The listing builds one solid part. Answer for the finished solid, in the listing's coordinates (mm). A direction names the side the tool comes from. Round coordinates to 2 decimals unless told otherwise and drop trailing zeros. Order: outer loops, then holes, each group sorted by start corner. A loop starts at its lowest first (then second) coordinate and runs counter-clockwise, first axis right, second up. Notation, with made-up numbers: (17.5, -26.5) - (64.5, -26.5) arc R26 cw to (64.5, -10.5) - close; hole circle Ø7 at (-5, 6.5). An arc over 180 degrees is marked (long way). One line per item, written item: value. Start each with the question number.
1. Flat-ended cylindrical pins translate along their axes: P1, Ø5, axis at x = -8, z = -16, coming from the +Y side (3 decimals); P2, Ø3, axis at x = -0.5, z = -17, coming from the -Y side; P3, Ø12, axis at x = -16, z = -20.5, coming from the -Y side; P4, Ø1, axis at y = -24, z = -27.5, coming from the +X side. Find the tip coordinate at first contact, or state that the pin passes through.
2. Section C-C, the plane z = -25 is taken. Give the vertices of the cut face in (x, y).
3. Straight lines are drawn through the part: line 1 (X direction, y = -24.5, z = -15.5); line 2 (Y direction, x = 30, z = -15); line 3 (Z direction, x = 1, y = -14). For each, find the intervals that lie inside material, in ascending order.
4. Section D-D, the plane z = -10.5 is taken. Give the vertices of the cut face in (x, y).
5. Section B-B, the plane y = 0 is taken. Give the vertices of the cut face in (x, z).
6. Section A-A, the plane x = -2 is taken. Give the vertices of the cut face in (y, z).
7. For a pull along Y with two mould halves and no side action, classify faces 1 (the cylindrical face through (27.675, -9.693, -10.846)), 2 (the flat face through (-0.5, -6.2, 0)), 3 (the cylindrical face through (-0.78, -5.95, -15.78)), 4 (the flat face through (-1, -13.016, -15)) as released by +Y, released by -Y, zero draft, split by the parting line, or undercut.
8. A tool of negligible diameter and unlimited length cuts with its end or side. For faces 5 (the flat face through (-30, -10, -11)), 6 (the flat face through (7.967, -24, -16)), 7 (the flat face through (24, 6, -22)), 8 (the cylindrical face through (-0.448, -21.128, -12.426)), from which of +Z, -Z, +X, -X, +Y, -Y can it reach the whole face along a straight path? Write none if from no direction.
from build123d import *

# Parameters (mm, degrees)
SKETCH1_R           = 6
BOSS_EXTRUDE1_DEPTH = 22
SKETCH3_R           = 3
CUT_EXTRUDE2_DEPTH  = 22
SKETCH4_R           = 6
BOSS_EXTRUDE2_DEPTH = 10
SKETCH5_R           = 3
CUT_EXTRUDE3_DEPTH  = 16


with BuildPart() as part:
    # Sketch1 → Boss-Extrude1 (new body)
    with BuildSketch(Plane.XY):
        with BuildLine():
            ThreePointArc((12.250598906, 10.291881579), (6.757584433, 14.502932553), (0, 16))
            ThreePointArc((0, 16), (-6.42506456, 14.653277633), (-11.768531852, 10.839818174))
            Line((-11.768531852, 10.839818174), (-13.649705535, 8.347786462))
            Line((-13.649705535, 8.347786462), (-26.599782678, -8.807462524))
            ThreePointArc((-26.599782678, -8.807462524), (-27.656705011, -9.685366602), (-28.994167614, -10))
            Line((-28.994167614, -10), (-32.032992561, -10))
            Line((-32.032992561, -10), (-32.032992561, -20.01649628))
            Line((-32.032992561, -20.01649628), (-27.5, -20.01649628))
            Line((-27.5, -20.01649628), (-8.032992561, -20.01649628))
            Line((-8.032992561, -20.01649628), (-8.032992561, -29.01649628))
            Line((-8.032992561, -29.01649628), (-0.032992561, -29.01649628))
            Line((-0.032992561, -29.01649628), (7.967007439, -29.01649628))
            Line((7.967007439, -29.01649628), (7.967007439, -20.01649628))
            Line((7.967007439, -20.01649628), (27.5, -20.01649628))
            Line((27.5, -20.01649628), (31.967007439, -20.01649628))
            Line((31.967007439, -20.01649628), (31.967007439, -10))
            Line((31.967007439, -10), (28.998198652, -10))
            ThreePointArc((28.998198652, -10), (27.65784727, -9.683925888), (26.599929469, -8.802305447))
            Line((26.599929469, -8.802305447), (13.293285189, 8.904412888))
            Line((13.293285189, 8.904412888), (12.250598906, 10.291881579))
        make_face()
        Circle(SKETCH1_R, mode=Mode.SUBTRACT)
    extrude(amount=-BOSS_EXTRUDE1_DEPTH)

    # Sketch3 → Cut-Extrude2 (cut)
    with BuildSketch(Plane(origin=(0, 0, 0), x_dir=(1, 0, 0), z_dir=(0, 1, 0))):
        with Locations(Location((0, 11.125223176, 0), (0, 0, 90))):
            Circle(SKETCH3_R)
    extrude(amount=CUT_EXTRUDE2_DEPTH, mode=Mode.SUBTRACT)

    # Sketch4 → Boss-Extrude2 (add)
    # profile 1 of 3: a face of its own
    with BuildSketch(Plane(origin=(0, 0, -22), x_dir=(-1, 0, 0), z_dir=(0, 0, -1))):
        with BuildLine():
            ThreePointArc((-12.250598906, 10.291881579), (-6.922536855, 14.424925771), (-0.364905179, 15.99583834))
            Line((-0.364905179, 15.99583834), (-32.361209339, 15.509505054))
            Line((-32.361209339, 15.509505054), (-31.967007439, -10))
            Line((-31.967007439, -10), (-28.998198652, -10))
            ThreePointArc((-28.998198652, -10), (-27.65784727, -9.683925888), (-26.599929469, -8.802305447))
            Line((-26.599929469, -8.802305447), (-12.250598906, 10.291881579))
        make_face()
    # profile 2 of 3: a face of its own
    with BuildSketch(Plane(origin=(0, 0, -22), x_dir=(-1, 0, 0), z_dir=(0, 0, -1))):
        with BuildLine():
            Line((31.626771502, 16.725648698), (-0.364905179, 15.99583834))
            ThreePointArc((-0.364905179, 15.99583834), (6.257540356, 14.725596378), (11.768531852, 10.839818174))
            Line((11.768531852, 10.839818174), (26.599782678, -8.807462524))
            ThreePointArc((26.599782678, -8.807462524), (27.656705011, -9.685366602), (28.994167614, -10))
            Line((28.994167614, -10), (32.032992561, -10))
            Line((32.032992561, -10), (31.626771502, 16.725648698))
        make_face()
    # profile 3 of 3: a face of its own
    with BuildSketch(Plane(origin=(0, 0, -22), x_dir=(-1, 0, 0), z_dir=(0, 0, -1))):
        with BuildLine():
            Line((32.032992561, -10), (28.994167614, -10))
            ThreePointArc((28.994167614, -10), (27.656705011, -9.685366602), (26.599782678, -8.807462524))
            Line((26.599782678, -8.807462524), (11.768531852, 10.839818174))
            ThreePointArc((11.768531852, 10.839818174), (-0.364905179, 15.99583834), (-12.250598906, 10.291881579))
            Line((-12.250598906, 10.291881579), (-26.599929469, -8.802305447))
            ThreePointArc((-26.599929469, -8.802305447), (-27.65784727, -9.683925888), (-28.998198652, -10))
            Line((-28.998198652, -10), (-31.967007439, -10))
            Line((-31.967007439, -10), (-31.967007439, -20.01649628))
            Line((-31.967007439, -20.01649628), (-7.967007439, -20.01649628))
            Line((-7.967007439, -20.01649628), (-7.967007439, -29.01649628))
            Line((-7.967007439, -29.01649628), (8.032992561, -29.01649628))
            Line((8.032992561, -29.01649628), (8.032992561, -20.01649628))
            Line((8.032992561, -20.01649628), (32.032992561, -20.01649628))
            Line((32.032992561, -20.01649628), (32.032992561, -10))
        make_face()
        with Locations(Location((0, 0, 0), (0, 0, 180))):
            Circle(SKETCH4_R, mode=Mode.SUBTRACT)
    extrude(amount=BOSS_EXTRUDE2_DEPTH)

    # Sketch5 → Cut-Extrude3 (cut)
    with BuildSketch(Plane.XZ.offset(29.01649628)):
        with Locations(Location((-0.579448602, -15.423300258, 0), (0, 0, 270))):
            Circle(SKETCH5_R)
    extrude(amount=-CUT_EXTRUDE3_DEPTH, mode=Mode.SUBTRACT)


solid = part.part
Answer list:
1. P1: stops at y = 15.025
1. P2: stops at y = -29.02
1. P3: stops at y = -20.02
1. P4: stops at x = 7.97
2. outline: (-32.03, -20.02) - (-8.03, -20.02) - (-8.03, -29.02) - (7.97, -29.02) - (7.97, -20.02) - (31.97, -20.02) - (31.97, -10) - (32.36, 15.51) - (0.36, 16) - (-31.63, 16.73) - (-32.03, -10) - close; hole circle Ø12 at (0, 0)
3. line 1: x = -8.03 to -3.58, 2.42 to 7.97
3. line 2: y = -20.02 to -10
3. line 3: z = -32 to -17.97, -12.87 to 0
4. outline: (-32.03, -20.02) - (-8.03, -20.02) - (-8.03, -29.02) - (7.97, -29.02) - (7.97, -20.02) - (31.97, -20.02) - (31.97, -10) - (29, -10) arc R3 cw to (26.6, -8.8) - (12.25, 10.29) arc R16 ccw to (2.93, 15.73) - (2.93, 5.23) arc R6 cw (long way) to (-2.93, 5.23) - (-2.93, 15.73) arc R16 ccw to (-11.77, 10.84) - (-26.6, -8.81) arc R3 cw to (-28.99, -10) - (-32.03, -10) - close
5. outline: (-31.88, -32) - (-6, -32) - (-6, 0) - (-19.95, 0) - (-19.95, -22) - (-31.88, -22) - close; (6, -32) - (32.12, -32) - (32.12, -22) - (19.98, -22) - (19.98, 0) - (6, 0) - close
6. outline: (-29.02, -32) - (-5.66, -32) - (-5.66, 0) - (-29.02, 0) - (-29.02, -12.78) - (-13.02, -12.78) - (-13.02, -18.07) - (-29.02, -18.07) - close; (5.66, -32) - (16.05, -32) - (16.05, -22) - (15.87, -22) - (15.87, -13.36) - (5.66, -13.36) - close; (5.66, -8.89) - (15.87, -8.89) - (15.87, 0) - (5.66, 0) - close
7. face 1: released by +Y
7. face 2: zero draft
7. face 3: undercut
7. face 4: released by -Y
8. face 5: +Z, -X, +Y
8. face 6: +Z, -Z, +X, -Y
8. face 7: +Z, +X, +Y
8. face 8: -Y
